The figure shows three views and two pictorial views of one solid part (mm, origin at its lowest corner). Answer the questions. A direction names the side the tool comes from. Give positions to 0.01 mm unless a question says otherwise; leave off trailing zeros. Order: outer loops, then holes, each group sorted by start corner. A loop starts at its lowest first (then second) coordinate and runs counter-clockwise, first axis right, second up. Notation, with made-up numbers: M 78.5,-28.5 L 129.5,-28.5 A8 ccw 129.5,-20.5 Z; hole C -14,-5 d5. An arc over 180 degrees is marked long. One line per item, written item: value. Start each with the question number.
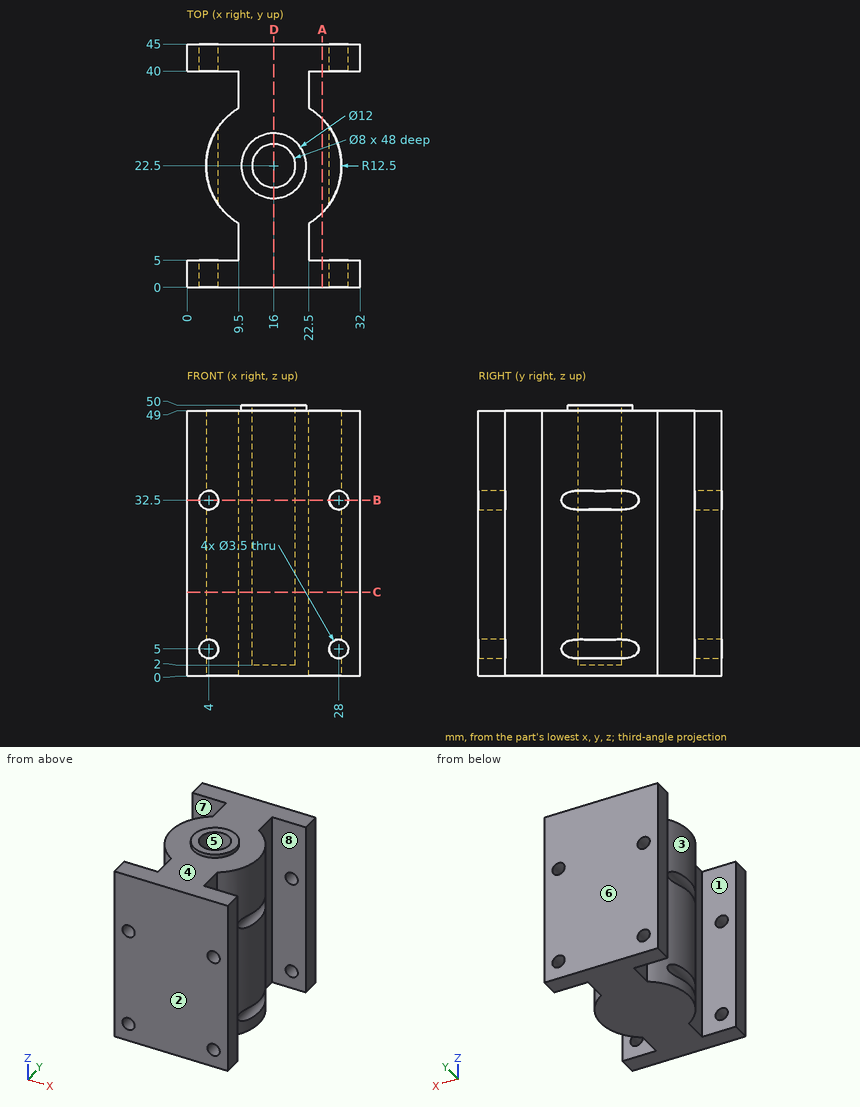
Q1. Each of these flat-tipped pins is pushed along its axis until it touches: pin 1 (12 mm diameter, centred on y = 27.5, z = 31.5, fed in from -X); pin 2 (5.5 mm diameter, centred on y = 10, z = 15.5, fed in from -X); pin 3 (8 mm diameter, centred on y = 11.5, z = 26, fed in from +X). Where does it stop, or does it pass through?
Q2. A tool of negligible diameter and unlimited length cuts with its end or side. For the marked faces 5, 6, 7 and 8, from which of +Z, -Z, +X, -X, +Y, -Y can it reach the whole face along a straight path? Write none if from no direction.
Q3. Find section C-C, the plane z = 15.5. Give the vertices of the cut face in (x, y), then the cut area to 3 significant figures.
Q4. Find section B-B, the plane z = 32.5. State how many separate pieces and enclosed holes the cut face has, then the cut area to 3 significant figures.
Q5. Find section A-A, the plane x = 25. Give the vertices of the cut face in (y, z).
Q6. Determine the mould class of the marked faces 1, 2, 3 and 4 for opening direction Y: released by +Y, released by -Y, zero draft, split by the parting line, or undercut.
Q7. Consider probe 1 along X at (y, z) = (41.5, 5); probe 2 along Y at (x, z) = (30, 45.5); probe 3 along Y at (x, z) = (9, 19). Determine where each line is inside the solid, lowest interval first.
Q8. Find section D-D, the plane x = 16. Give the vertices of the cut face in (y, z).
Evaluation:
1. pin 1: x = 3.5
1. pin 2: x = 8.18
1. pin 3: x = 26.36
2. face 5: +Z
2. face 6: +Z, -Z, +X, -X, +Y
2. face 7: +Z, -Z, -X
2. face 8: +Z, -Z, +X
3. outline: M 0,0 L 32,0 L 32,5 L 22.5,5 L 22.5,11.82 A12.5 ccw 22.5,33.18 L 22.5,40 L 32,40 L 32,45 L 0,45 L 0,40 L 9.5,40 L 9.5,33.18 A12.5 ccw 9.5,11.82 L 9.5,5 L 0,5 Z; hole C 16,22.5 d8
3. area: 906 mm2
4. separate pieces: 5
4. enclosed holes: 1
4. area: 792 mm2
5. outline: M 0,0 L 5,0 L 5,49 L 0,49 Z; M 13.83,0 L 31.17,0 L 31.17,49 L 13.83,49 Z; M 40,0 L 45,0 L 45,49 L 40,49 Z
6. face 1: undercut
6. face 2: released by -Y
6. face 3: undercut
6. face 4: zero draft
7. probe 1: 0 to 2.25, 5.75 to 26.25, 29.75 to 32
7. probe 2: 0 to 5, 40 to 45
7. probe 3: 0 to 5, 12.14 to 32.86, 40 to 45
8. outline: M 0,0 L 45,0 L 45,49 L 28.5,49 L 28.5,50 L 26.5,50 L 26.5,2 L 18.5,2 L 18.5,50 L 16.5,50 L 16.5,49 L 0,49 Z
